```python
from build123d import *

# Parameters (mm, degrees)
CROQUIS1_R              = 10
CROQUIS1_R_2            = 6
SALIENTE_EXTRUIR1_DEPTH = 10
CROQUIS2_R              = 4.5
CORTAR_EXTRUIR1_DEPTH   = 10
CHAFL_N1_DEPTH          = 10
CROQUIS3_W              = 7
CROQUIS3_H              = 3
SALIENTE_EXTRUIR2_DEPTH = 10
CROQUIS4_R              = 1.675
CORTAR_EXTRUIR2_DEPTH   = 10
REDONDEO2_R             = 4
CORTAR_EXTRUIR3_DEPTH   = 3.5


with BuildPart() as part:
    # Croquis1 → Saliente-Extruir1 (new body)
    # profile 1 of 2: a face of its own
    with BuildSketch(Plane(origin=(0, 0, 0), x_dir=(1, 0, 0), z_dir=(0, 1, 0))):
        Circle(CROQUIS1_R)
        with Locations(Location((0, 0, 0), (0, 0, 270))):
            Circle(CROQUIS1_R_2, mode=Mode.SUBTRACT)
    # profile 2 of 2: a face of its own
    with BuildSketch(Plane(origin=(0, 0, 0), x_dir=(1, 0, 0), z_dir=(0, 1, 0))):
        with BuildLine():
            Line((-13.5, 16), (-4.582575695, 16))
            ThreePointArc((-4.582575695, 16), (0, 13), (4.582575695, 16))
            Line((4.582575695, 16), (13.5, 16))
            Line((13.5, 16), (13.5, 6))
            Line((13.5, 6), (-13.5, 6))
            Line((-13.5, 6), (-13.5, 16))
        make_face()
    extrude(amount=SALIENTE_EXTRUIR1_DEPTH)

    # Croquis2 → Cortar-Extruir1 (cut)
    with BuildSketch(Plane(origin=(0, 10, 0), x_dir=(1, 0, 0), z_dir=(0, 1, 0))):
        with Locations(Location((-7.5, 10.5, 0), (0, 0, 270))):
            Circle(CROQUIS2_R)
        with Locations(Location((7.5, 10.5, 0), (0, 0, 270))):
            Circle(CROQUIS2_R)
    extrude(amount=-CORTAR_EXTRUIR1_DEPTH, mode=Mode.SUBTRACT)

    # Chaflán1: read off the stored shape, not the designer's step
    # Chaflán1 outline → Chaflán1 (add)
    with BuildSketch(Plane(origin=(0, 0, 0), x_dir=(1, 0, 0), z_dir=(0, 1, 0))):
        with BuildLine():
            ThreePointArc((8, 6), (9.633249581, 2.68337521), (9.949874371, -1))
            Line((9.949874371, -1), (11.371284996, 6))
            Line((11.371284996, 6), (8, 6))
        make_face()
        with BuildLine():
            Line((-11.371284996, 6), (-9.949874371, -1))
            ThreePointArc((-9.949874371, -1), (-9.633249581, 2.68337521), (-8, 6))
            Line((-8, 6), (-11.371284996, 6))
        make_face()
    extrude(amount=CHAFL_N1_DEPTH)

    # Croquis3 → Saliente-Extruir2 (add)
    with BuildSketch(Plane(origin=(0, 0, 0), x_dir=(1, 0, 0), z_dir=(0, 1, 0))):
        with Locations((0, -10)):
            Rectangle(CROQUIS3_W, CROQUIS3_H)
    extrude(amount=SALIENTE_EXTRUIR2_DEPTH)

    # Croquis4 → Cortar-Extruir2 (cut)
    with BuildSketch(Plane.XY.offset(11.5)):
        with Locations((0, 5)):
            Circle(CROQUIS4_R)
    extrude(amount=-CORTAR_EXTRUIR2_DEPTH, mode=Mode.SUBTRACT)

    # Redondeo2
    # the kernel refuses this fillet: 4 mm, written as the material it adds along each edge
    with BuildSketch(Plane(origin=(-3.5, 10, 9.367496998), x_dir=(-0.8956592986601979, 0, -0.4447408467001005), z_dir=(0, -1, 0))) as redondeo2_piece_1:
        with BuildLine():
            CenterArc((2.475122402, -3.978671502), REDONDEO2_R, 95.919444292, 52.938021971)
            Line((-0.948411191, -1.909996144), (-1.016881863, -1.868622636))
            ThreePointArc((-1.016881863, -1.868622636), (-0.545858339, -0.919418804), (-0.071652744, 0.035579268))
            Line((-0.071652744, 0.035579268), (0.008250408, 0.07957343))
            ThreePointArc((0.008250408, 0.07957343), (1.031301001, 0.026678755), (2.054351594, 0.07957343))
            Line((2.054351594, 0.07957343), (2.062602002, 0))
        make_face()
    extrude(amount=10)
    with BuildSketch(Plane(origin=(3.5, 10, 9.367496998), x_dir=(0, 0, 1), z_dir=(0, -1, 0))) as redondeo2_piece_2:
        with BuildLine():
            CenterArc((2.462746094, -3.986344127), REDONDEO2_R, 94.735774331, 52.938021971)
            Line((-0.917323361, -1.847388662), (-0.98492475, -1.804609553))
            ThreePointArc((-0.98492475, -1.804609553), (-0.482556755, -0.911829199), (-0.074939976, 0.028))
            Line((-0.074939976, 0.028), (0, 0.08))
            ThreePointArc((0, 0.08), (1.066251501, 0.08), (2.125898141, 0.079726883))
            Line((2.125898141, 0.079726883), (2.132503002, 0))
        make_face()
    extrude(amount=10)
    # the kernel refuses this fillet: 4 mm, written as the material it takes off along each edge
    with BuildSketch(Plane(origin=(13.5, -10, -16), x_dir=(-1, 0, 0), z_dir=(0, 1, 0)), Plane(origin=(-13.5, -10, -16), x_dir=(0, 0, 1), z_dir=(0, 1, 0))) as redondeo2_2_piece_1:
        with BuildLine():
            CenterArc((REDONDEO2_R, REDONDEO2_R), REDONDEO2_R, 180, 90)
            Line((0, REDONDEO2_R), (-REDONDEO2_R * 0.02, REDONDEO2_R))
            Line((-REDONDEO2_R * 0.02, REDONDEO2_R), (-REDONDEO2_R * 0.02, -REDONDEO2_R * 0.02))
            Line((-REDONDEO2_R * 0.02, -REDONDEO2_R * 0.02), (REDONDEO2_R, -REDONDEO2_R * 0.02))
            Line((REDONDEO2_R, -REDONDEO2_R * 0.02), (REDONDEO2_R, 0))
        make_face()
    extrude(amount=30, mode=Mode.SUBTRACT)
    with BuildSketch(Plane(origin=(13.5, -8.838231039, -6), x_dir=(0, 0, -1), z_dir=(0, 1, 0))) as redondeo2_2_piece_2:
        with BuildLine():
            CenterArc((3.535292416, 4), REDONDEO2_R, 207.892961789, 62.107038211)
            Line((0, 2.128715004), (-0.070705848, 2.091289304))
            ThreePointArc((-0.070705848, 2.091289304), (-0.08, 1.064357502), (-0.08, 0))
            Line((-0.08, 0), (0, -0.08))
            Line((0, -0.08), (3.535292416, -0.08))
            Line((3.535292416, -0.08), (3.535292416, 0))
        make_face()
    extrude(amount=27.676462078, mode=Mode.SUBTRACT)
    with BuildSketch(Plane(origin=(-13.5, -8.838231039, -6), x_dir=(1, 0, 0), z_dir=(0, 1, 0))) as redondeo2_2_piece_3:
        with BuildLine():
            CenterArc((4, 3.535292416), REDONDEO2_R, 180, 62.107038211)
            Line((0, 3.535292416), (-0.08, 3.535292416))
            Line((-0.08, 3.535292416), (-0.08, 0))
            Line((-0.08, 0), (0, -0.08))
            ThreePointArc((0, -0.08), (1.064357502, -0.08), (2.091289304, -0.070705848))
            Line((2.091289304, -0.070705848), (2.128715004, 0))
        make_face()
    extrude(amount=27.676462078, mode=Mode.SUBTRACT)
    with BuildSketch(Plane(origin=(4.582575695, -5.314070594, -16), x_dir=(-0.5401558180759948, 0, 0.8415650255319863), z_dir=(0, 1, 0))) as redondeo2_2_piece_4:
        with BuildLine():
            CenterArc((2.218089643, 3.949477654), REDONDEO2_R, 212.694246687, 48.189685104)
            Line((-1.14817046, 1.788854382), (-1.215495662, 1.745641917))
            Line((-1.215495662, 1.745641917), (-0.067325202, -0.043212465))
            Line((-0.067325202, -0.043212465), (0.012674798, -0.078989553))
            ThreePointArc((0.012674798, -0.078989553), (0.792174872, -0.016847068), (1.571674947, -0.078989553))
            Line((1.571674947, -0.078989553), (1.584349745, 0))
        make_face()
    extrude(amount=20.628141188, mode=Mode.SUBTRACT)
    with BuildSketch(Plane(origin=(-4.582575695, -5.314070594, -16), x_dir=(-1, 0, 0), z_dir=(0, 1, 0))) as redondeo2_2_piece_5:
        with BuildLine():
            CenterArc((2.125628238, 4), REDONDEO2_R, 221.810314896, 48.189685104)
            Line((-0.855795732, 1.333333333), (-0.915424212, 1.28))
            ThreePointArc((-0.915424212, 1.28), (-0.442075769, 0.657566625), (-0.073321211, -0.032))
            Line((-0.073321211, -0.032), (0, -0.08))
            Line((0, -0.08), (2.125628238, -0.08))
            Line((2.125628238, -0.08), (2.125628238, 0))
        make_face()
    extrude(amount=20.628141188, mode=Mode.SUBTRACT)

    # Croquis5 → Cortar-Extruir3 (cut)
    with BuildSketch(Plane.XY.offset(11.5)):
        Polygon((4.907477288, 5), (2.453738644, 9.25), (-2.453738644, 9.25), (-4.907477288, 5), (-2.453738644, 0.75), (2.453738644, 0.75), align=None)
    extrude(amount=-CORTAR_EXTRUIR3_DEPTH, mode=Mode.SUBTRACT)


solid = part.part
```
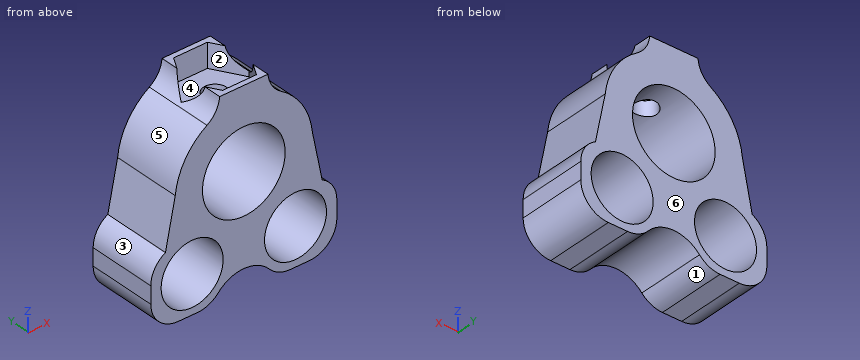
Can you work these out from the model? Positions are in its coordinate system, mm. Face numbers are marked on the shaded views. A direction names the side the tool comes from. Round coordinates to 2 decimals unless told otherwise and drop trailing zeros. Loops run counter-clockwise (first coordinate to the right, second up) from the corner with the lowest first, then second, coordinate; pieces in that order, holes last.
Item 1: Suppose I cut it at A-A, the plane x = 0. Write out the boundary of the cut face in (y, z) (3 decimals), then the cut area to 4 significant figures.
Item 2: Will these pins go through, and if not, where does the flat tip stop? pin 1 Ø14 at (x, z) = (0, 0) entering from +Y; pin 2 Ø2.5 at (x, y) = (-2, 6.5) entering from +Z; pin 3 Ø2 at (y, z) = (7.5, -6.5) entering from -X; pin 4 Ø5.5 at (x, y) = (0, 5) entering from -Z.
Item 3: Please list where these lines run through material, in increasing order: L1, parallel to X at y = 5.25, z = -10.5; L2, parallel to Z at x = -4, y = 4.75; L3, parallel to Z at x = 5.5, y = 6.5.
Item 4: Suppose I cut it at C-C, the plane z = -10.5. Write out the boundary of the cut face in (x, y).
Item 5: Suppose I cut it at D-D, the plane y = 8. Write out the boundary of the cut face in (x, z), then the cut area to 3 significant figures.
Item 6: Suppose I cut it at B-B, the plane z = 3.25. Write out the boundary of the cut face in (x, y), then the cut area to 3 significant figures.
Item 7: If we mould it in two halves opening along Y, with no side actions, what happens to the marked faces 4, 5 and 6? For each: +Y half, -Y half, draft (parallel to the pull), parting line (faces both ways), or undercut.
Item 8: Which directions (+Z, -Z, +X, -X, +Y, -Y) give clear straight access to the entire face, cutting with the end or side of a thin tool? Please do the marked faces 1, 2 and 3.
Reported:
1. outline: (0, -13) - (10, -13) - (10, -6) - (0, -6) - close; (0, 6) - (3.325, 6) - (3.325, 8) - (0.75, 8) - (0.75, 11.5) - (0, 11.5) - close; (6.675, 6) - (10, 6) - (10, 11.5) - (9.25, 11.5) - (9.25, 8) - (6.675, 8) - close
1. area: 88.55 mm2
2. pin 1: stops at y = 10
2. pin 2: stops at z = 8
2. pin 3: stops at x = -12.94
2. pin 4: stops at z = -13.82
3. L1: x = -13.5 to -12, -3 to 3, 12 to 13.5
3. L2: z = -14.94 to -13.33, -7.67 to -4.47, 4.47 to 8
3. L3: z = -15.81 to -14.53, -6.47 to -2.4, 2.4 to 8.35
4. outline: (-13.5, 0) - (-12, 0) - (-12, 10) - (-13.5, 10) - close; (-3, 0) - (3, 0) - (3, 10) - (-3, 10) - close; (12, 0) - (13.5, 0) - (13.5, 10) - (12, 10) - close
5. outline: (-13.5, -12) arc R4 ccw to (-9.5, -16) - (-6.71, -16) arc R4 ccw to (-3.73, -14.67) arc R5 cw to (3.73, -14.67) arc R4 ccw to (6.71, -16) - (9.5, -16) arc R4 ccw to (13.5, -12) - (13.5, -9.54) arc R4 ccw to (11.37, -6) - (9.95, 1) arc R10 ccw to (5.35, 8.45) arc R4 cw to (3.5, 11.5) - (3.18, 11.5) - (3.18, 8) - (-3.18, 8) - (-3.18, 11.5) - (-3.5, 11.5) arc R4 cw to (-5.35, 8.45) arc R10 ccw to (-9.95, 1) - (-11.37, -6) arc R4 ccw to (-13.5, -9.54) - close; hole circle Ø9 at (-7.5, -10.5); hole circle Ø12 at (0, 0); hole circle Ø9 at (7.5, -10.5)
5. area: 275 mm2
6. outline: (-9.46, 0) - (-5.04, 0) - (-5.04, 10) - (-9.46, 10) - close; (5.04, 0) - (9.46, 0) - (9.46, 10) - (5.04, 10) - close
6. area: 88.3 mm2
7. face 4: undercut
7. face 5: draft
7. face 6: +Y half
8. face 1: -Z, +Y, -Y
8. face 2: +Z
8. face 3: +Z, -X, +Y, -Y
